```python
from build123d import *

# Parameters (mm, degrees)
SKETCH1_R           = 1.6
BOSS_EXTRUDE1_DEPTH = 12


with BuildPart() as part:
    # Sketch1 → Boss-Extrude1 (new body)
    with BuildSketch(Plane.XY):
        with BuildLine():
            ThreePointArc((-3.75, 2.523123532), (0, 6.273123532), (-3.75, 10.023123532))
            Line((-3.75, 10.023123532), (-8.75, 10.023123532))
            Line((-8.75, 10.023123532), (-8.75, -2.792382112))
            Line((-8.75, -2.792382112), (38.25, -2.792382112))
            Line((38.25, -2.792382112), (38.25, 10.023123532))
            Line((38.25, 10.023123532), (33.25, 10.023123532))
            ThreePointArc((33.25, 10.023123532), (29.5, 6.273123532), (33.25, 2.523123532))
            Line((33.25, 2.523123532), (29.5, 2.523123532))
            Line((29.5, 2.523123532), (29.5, 0))
            Line((29.5, 0), (0, 0))
            Line((0, 0), (0, 2.523123532))
            Line((0, 2.523123532), (-3.75, 2.523123532))
        make_face()
        with Locations(Location((-3.75, 6.273123532, 0), (0, 0, 180))):
            Circle(SKETCH1_R, mode=Mode.SUBTRACT)
        with Locations(Location((33.25, 6.273123532, 0), (0, 0, 180))):
            Circle(SKETCH1_R, mode=Mode.SUBTRACT)
    extrude(amount=BOSS_EXTRUDE1_DEPTH)


solid = part.part
```
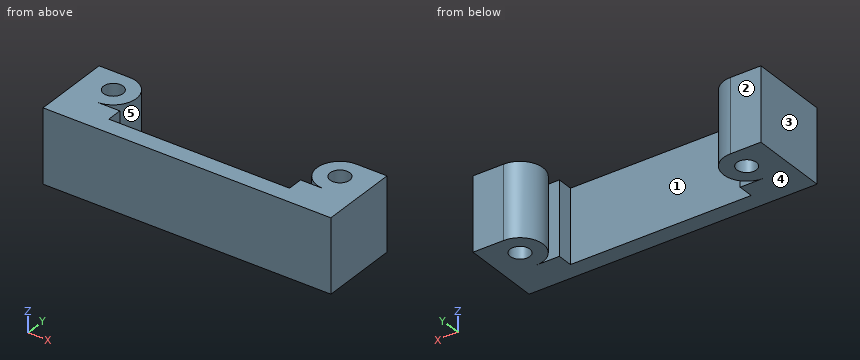
CAD build for the part. Positions are in the model's coordinates, mm. Face numbers are marked on the shaded views. A direction names the side the tool comes from. Round coordinates to 2 decimals unless told otherwise and drop trailing zeros. Write each loop counter-clockwise with the first axis right and the second up, starting at its lowest first coordinate (ties: lowest second). Pieces come first, ordered by that corner, then holes.
Item 1: Band-saw the part on D-D on x = 22. Write the cut outline in (y, z).
Filled in:
outline: (-2.79, 0) - (0, 0) - (0, 12) - (-2.79, 12) - close
Item 2: Tool access for the marked faces 1 and 2: list every direction of +Z, -Z, +X, -X, +Y, -Y with a clear straight run to the whole face (end or side of a thin tool).
Filled in:
face 1: +Z, -Z, +Y
face 2: +Z, -Z, +X, -X, +Y
Item 3: Drill centre lines: L1, parallel to X at y = 1.25, z = 8.25; L2, parallel to Y at x = 33.5, z = 11.5; L3, parallel to Y at x = 28.5, z = 11. Where is each one in solid material? Low to high.
Filled in:
L1: x = -8.75 to 0, 29.5 to 38.25
L2: y = -2.79 to 4.69, 7.85 to 10.02
L3: y = -2.79 to 0
Item 4: Mould opens along X. For the marked faces 3, 4 and 5 say: released by +X, released by -X, zero draft, split by the parting line, or undercut.
Filled in:
face 3: released by -X
face 4: zero draft
face 5: undercut
Item 5: Drop flat-ended pins along their axis: pin 1 Ø2 at (x, z) = (25.5, 5.5) entering from +Y; pin 2 Ø3 at (x, z) = (-2, 5) entering from +Y. Give the stop position or say it passes through.
Filled in:
pin 1: stops at y = 0
pin 2: stops at y = 10.01
Item 6: Band-saw the part on A-A on y = 2. Write the cut outline in (x, z).
Filled in:
outline: (-8.75, 0) - (0, 0) - (0, 12) - (-8.75, 12) - close; (29.5, 0) - (38.25, 0) - (38.25, 12) - (29.5, 12) - close
Item 7: Band-saw the part on B-B on z = 10.25. Write the cut outline in (x, y), then the cut area to 3 significant figures.
Filled in:
outline: (-8.75, -2.79) - (38.25, -2.79) - (38.25, 10.02) - (33.25, 10.02) arc R3.75 ccw to (33.25, 2.52) - (29.5, 2.52) - (29.5, 0) - (0, 0) - (0, 2.52) - (-3.75, 2.52) arc R3.75 ccw to (-3.75, 10.02) - (-8.75, 10.02) - close; hole circle Ø3.2 at (-3.75, 6.27); hole circle Ø3.2 at (33.25, 6.27)
area: 278 mm2
Item 8: Band-saw the part on C-C on x = 30.5. Write the cut outline in (y, z).
Filled in:
outline: (-2.79, 0) - (2.52, 0) - (2.52, 12) - (-2.79, 12) - close; (3.72, 0) - (8.82, 0) - (8.82, 12) - (3.72, 12) - close
